```python
from build123d import *

# Parameters (mm, degrees)
F0_W     = 50
F0_H     = 50
F1_DEPTH = 25
F2_T     = -2.5
F3_T     = 2.5


# Not quite as in the source:
# - a shell that OpenCascade refuses in one call is made with other operations: the cavity is built on its own and cut out


with BuildPart() as f1:
    # F0 (on Top) → F1 (new body)
    with BuildSketch(Plane.XY):
        with Locations((0.357497856, 6.2575038522)):
            Rectangle(F0_W, F0_H)
    extrude(amount=F1_DEPTH)

    # F2
    f2_openings = [f1.faces().sort_by_distance(p)[0] for p in [
        (0.357498, 6.257504, 25),
        (0.357498, 6.257504, 0),
    ]]
    offset(amount=F2_T, openings=f2_openings)

    # F3: shell of thickness 2.5, made by hand


with BuildPart() as f3_core1:
    # F3_t2: copy of F1
    add(f1.part)

    # the walls: a layer under each face that stays
    f3_faces = [f3_core1.faces().sort_by_distance(p)[0] for p in [
        (0.357497856, -18.7424961478, 12.5),
        (-22.9758354773, -17.0758294811, 0),
        (-22.142502144, 6.2575038522, 12.5),
    ]]
    thicken(f3_faces, amount=-F3_T, mode=Mode.SUBTRACT)


with BuildPart() as f1_1:
    add(f1.part)

    # what is left inside the walls is the cavity
    f3_cavity = [f3_core1.part.solids().sort_by_distance(p)[0] for p in [
        (0.357498, 31.232504, 17.5),
    ]]
    add(f3_cavity, mode=Mode.SUBTRACT)


solid = f1_1.part
```
Geometry: final body of the model. Coordinates: model frame, mm. A direction names the side the tool comes from. Round coordinates to 2 decimals unless told otherwise and drop trailing zeros. Order: outer loops, then holes, each group sorted by start corner. A loop starts at its lowest first (then second) coordinate and runs counter-clockwise, first axis right, second up. Notation, with made-up numbers: (17.5, -4.5) - (31.5, -4.5) arc R15 cw to (31.5, 14.5) - close; hole circle Ø10 at (34, 9). An arc over 180 degrees is marked (long way). Use CSV: the item, a comma, the result in double quotes. Start each with the question number.
Q1. Section query A-A (x = 21.5). Return loops of the section in (y, z), and give its area (4 significant figures).
Q2. Section query B-B (y = -0.5). Return loops of the section in (x, z), and give its area (4 significant figures).
Q3. Section query C-C (z = 20). Return loops of the section in (x, y), and give its area (4 significant figures).
Q4. Material intervals for line 1 along X through (y, z) = (-14.5, 1.5); line 2 along Y through (x, z) = (-10, 2); line 3 along X through (y, z) = (5.5, 11.25), sorted ascending. Write a range as from..to.
Q5. Access query for faces 4 (the face through (0, 28.758, 1)), 5 (the face through (-23, 28.758, 14)), 6 (the face through (-11, -18, 25)), 7 (the face through (11, 30, 2.5)). Directions: +Z, -Z, +X, -X, +Y, -Y. A direction counts if a zero-diameter tool reaches every point of the face in a straight line with its end or side. Return the directions, or none.
Q6. Mould query, pull axis X, two halves, no side actions, for faces 1 (the face through (-24.643, 6, 12)), 2 (the face through (-2, -18, 0)), 3 (the face through (22.857, 6, 1)). Classes: +X half, -X half, draft (parallel to the pull), parting line (faces both ways), or undercut.
Q7. First-contact query: pin 1 (12 mm diameter, centred on x = -2.5, y = 20.5, fed in from +Z); pin 2 (1.2 mm diameter, centred on x = -24, z = 16.5, fed in from +Y); pin 3 (8 mm diameter, centred on x = 4, z = 19.5, fed in from +Y); pin 4 (10 mm diameter, centred on y = 8.5, z = 19, fed in from +X). Flat tips, straight axial feed; report the tip coordinate or a pass-through.
Result set:
1,outline,"(-18.74, 0) - (-16.24, 0) - (-16.24, 25) - (-18.74, 25) - close; (28.76, 0) - (31.26, 0) - (31.26, 2.5) - (28.76, 2.5) - close"
1,area,"68.75 mm2"
2,outline,"(-24.64, 0) - (-22.14, 0) - (-22.14, 25) - (-24.64, 25) - close; (22.86, 0) - (25.36, 0) - (25.36, 2.5) - (22.86, 2.5) - close"
2,area,"68.75 mm2"
3,outline,"(-24.64, -18.74) - (25.36, -18.74) - (25.36, -16.24) - (-22.14, -16.24) - (-22.14, 28.76) - (-24.64, 28.76) - close"
3,area,"237.5 mm2"
4,line 1,"x = -24.64..-22.14, 22.86..25.36"
4,line 2,"y = -18.74..-16.24, 28.76..31.26"
4,line 3,"x = -24.64..-22.14"
5,face 4,"+Z, -Z"
5,face 5,"+Z, +X, -X, +Y"
5,face 6,"+Z, +X, -X, +Y, -Y"
5,face 7,"+Z, +X, +Y"
6,face 1,"-X half"
6,face 2,"draft"
6,face 3,"undercut"
7,pin 1,"passes through"
7,pin 2,"stops at y = 28.76"
7,pin 3,"stops at y = -16.24"
7,pin 4,"stops at x = -22.14"
